The listing builds one solid part. Answer for the finished solid, in the listing's coordinates (mm). A direction names the side the tool comes from. Round coordinates to 2 decimals unless told otherwise and drop trailing zeros. Order: outer loops, then holes, each group sorted by start corner. A loop starts at its lowest first (then second) coordinate and runs counter-clockwise, first axis right, second up. Notation, with made-up numbers: M 45,12 L 87,12 A27 ccw 87,42 Z; hole C 61.25,6 d2. An arc over 180 degrees is marked long. Put each result on its own line as item: value. Start each with the question number.
1. The mould has two halves that part along X. Classify faces 1 (the face through (0, 10, 30)), 2 (the face through (-51, -1, 15)), 3 (the face through (-1, -1, 0)): +X half, -X half, draft (parallel to the pull), parting line (faces both ways), or undercut.
2. The part is cut by section B-B (x = -21). Give the vertices of the cut face in (y, z), then the cut area to 3 significant figures.
3. The part is cut by section C-C (y = 27). Give the vertices of the cut face in (x, z), then the cut area to 3 significant figures.
4. Which of the six approach directions +Z, -Z, +X, -X, +Y, -Y give full straight-line access (tool end or side, diameter ignored) to faces 4 (the face through (50.3, -41.622, 13.4)), 5 (the face through (-1, -1, -1)), 6 (the face through (-1, 75, 15))?
5. The part is cut by section A-A (z = 10.5). Give the vertices of the cut face in (x, y).
6. Consider line 1 (X direction, y = 10, z = 26); line 2 (Y direction, x = -20, z = 2); line 3 (Y direction, x = 32.5, z = 16). Determine where each line is inside the solid, lowest interval first.
7. Each of these flat-tipped pins is pushed along its axis until it touches: pin 1 Ø0.8 at (y, z) = (-55.5, -0.5) entering from +X; pin 2 Ø1.2 at (x, y) = (34.5, 59) entering from +Z. Where does it stop, or does it pass through?
8. The part is cut by section D-D (z = 27.5). Give the vertices of the cut face in (x, y).
from build123d import *

# Parameters (mm, degrees)
SKETCH_1_W           = 102
SKETCH_1_H           = 152
SKETCH_1_W_2         = 100
SKETCH_1_H_2         = 150
EXTRUDE_1_DEPTH      = 30
EXTRUDE_2_DEPTH      = 76
EXTRUDE_2_DEPTH_BACK = 76
SKETCH_2_W           = 102
SKETCH_2_H           = 1
SKETCH_3_R           = 9.5
EXTRUDE_3_DEPTH      = 30
EXTRUDE_4_DEPTH      = 15
SKETCH_6_W           = 31
SKETCH_6_H           = 33.017960066
CUT_EXTRUDE_1_DEPTH  = 3
EXTRUDE_5_DEPTH      = 31


with BuildPart() as part:
    # 草图1 → 凸台-拉伸1 (new body)
    with BuildSketch(Plane.XY):
        Rectangle(SKETCH_1_W, SKETCH_1_H)
        Rectangle(SKETCH_1_W_2, SKETCH_1_H_2, mode=Mode.SUBTRACT)
    extrude(amount=EXTRUDE_1_DEPTH)

    # 草图2 → 凸台-拉伸2 (add, two sides: drawn at the far end of the back side and taken through both)
    with BuildSketch(Plane(origin=(0, 0, 0), x_dir=(1, 0, 0), z_dir=(0, 1, 0)).offset(-EXTRUDE_2_DEPTH_BACK)):
        with Locations((0, 0.5)):
            Rectangle(SKETCH_2_W, SKETCH_2_H)
    extrude(amount=EXTRUDE_2_DEPTH + EXTRUDE_2_DEPTH_BACK)

    # 草图3 → 凸台-拉伸3 (add)
    with BuildSketch(Plane.XY):
        with Locations((0, 9.764589886)):
            Circle(SKETCH_3_R)
    extrude(amount=EXTRUDE_3_DEPTH)

    # 草图5 → 凸台-拉伸4 (add)
    with BuildSketch(Plane.XY):
        with BuildLine():
            ThreePointArc((36, 59), (35.414213562, 60.414213562), (34, 61))
            Line((34, 61), (34, 59))
            Line((34, 59), (36, 59))
        make_face()
        with BuildLine():
            Line((34, 59), (34, 61))
            ThreePointArc((34, 61), (32.585786438, 57.585786438), (36, 59))
            Line((36, 59), (34, 59))
        make_face()
    extrude(amount=EXTRUDE_4_DEPTH)

    # 草图6 → 切除-拉伸1 (cut)
    with BuildSketch(Plane(origin=(51, 0, 0), x_dir=(0, 0, -1), z_dir=(1, 0, 0))):
        with Locations((-14.5, -58.131256351)):
            Rectangle(SKETCH_6_W, SKETCH_6_H)
    extrude(amount=-CUT_EXTRUDE_1_DEPTH, mode=Mode.SUBTRACT)

    # 草图7 → 凸台-拉伸5 (add)
    with BuildSketch(Plane.XY.offset(30)):
        Polygon((49.826203417, -75.312750473), (51, -75.320118192), (0, -35.235410114), (0, -36.150616776), align=None)
    extrude(amount=-EXTRUDE_5_DEPTH)


solid = part.part
Resolved:
1. face 1: draft
1. face 2: -X half
1. face 3: undercut
2. outline: M -76,-1 L 76,-1 L 76,30 L 75,30 L 75,0 L -75,0 L -75,30 L -76,30 Z
2. area: 212 mm2
3. outline: M -51,-1 L 51,-1 L 51,30 L 50,30 L 50,0 L -50,0 L -50,30 L -51,30 Z
3. area: 162 mm2
4. face 4: +Z, -Z, +X
4. face 5: -Z, +X, -X, +Y, -Y
4. face 6: +Z
5. outline: M -51,-76 L 51,-76 L 51,-74.64 L 50.13,-74.64 L 0,-35.24 L 0,-36.15 L 49.43,-75 L -50,-75 L -50,75 L 50,75 L 50,-41.62 L 51,-41.62 L 51,76 L -51,76 Z; C 0,9.76 d19; C 34,59 d4
6. line 1: -51 to -50, -9.5 to 9.5, 50 to 51
6. line 2: -76 to -75, 75 to 76
6. line 3: -76 to -75, -61.69 to -60.78, 75 to 76
7. pin 1: x = 48
7. pin 2: z = 15
8. outline: M -51,-76 L 51,-76 L 51,-74.64 L 50.13,-74.64 L 0,-35.24 L 0,-36.15 L 49.43,-75 L -50,-75 L -50,75 L 50,75 L 50,-41.62 L 51,-41.62 L 51,76 L -51,76 Z; C 0,9.76 d19
